CAD build for the part. Positions are in the model's coordinates, mm. A direction names the side the tool comes from. Coordinates: 2 decimals unless noted, no trailing zeros. Loops run counter-clockwise (first coordinate to the right, second up) from the corner with the lowest first, then second, coordinate; pieces in that order, holes last. Notation, with made-up numbers: (2, 27) -> (40, 27) arc R23 ccw to (40, 61) -> close; hole circle Ø6 at (28, 69.25). An arc over 180 degrees is marked (long way). Answer as CSV lines item,"result". Start each with the question number.
```python
from build123d import *

# Parameters (mm, degrees)
BOSS_EXTRUDE1_DEPTH = 40
SKETCH2_R           = 2.5
CUT_EXTRUDE1_DEPTH  = 79.89866919


with BuildPart() as part:
    # Sketch1 → Boss-Extrude1 (new body)
    with BuildSketch(Plane(origin=(0, 0, 0), x_dir=(1, 0, 0), z_dir=(0, 1, 0))):
        Polygon((0, 0), (0, 20), (3, 20), (3, 3), (65, 3), (65, 0), align=None)
    extrude(amount=BOSS_EXTRUDE1_DEPTH)

    # Sketch2 → Cut-Extrude1 (cut, through all)
    with BuildSketch(Plane.XY):
        with Locations((21.15, 20)):
            Circle(SKETCH2_R)
        with Locations((57.65, 20)):
            Circle(SKETCH2_R)
    extrude(amount=-CUT_EXTRUDE1_DEPTH, mode=Mode.SUBTRACT)


solid = part.part
```
Q1. Saw through at B-B (x = 21.15). List the corners of the cut face in (y, z).
Q2. Probe probe 1 along Y at (x, z) = (21.15, -2.1); probe 2 along Z at (x, y) = (40, 9); probe 3 along X at (y, z) = (36, -11). List the from-to ranges inside material, lowest first. Write a range as from..to.
Q3. Which spindle directions (+Z, -Z, +X, -X, +Y, -Y) get a long thin tool onto all of the face, cutting with end or side? Do faces 4 (the flat face through (3, 20, -12)), 5 (the cylindrical face through (58.99, 22.11, -1.48)). Say none if no direction does.
Q4. Saw through at A-A (y = 20). List the corners of the cut face in (x, z).
Q5. Saw through at C-C (y = 12.5). List the corners of the cut face in (x, z), and give its area (3 significant figures).
Q6. Saw through at D-D (z = -6.5). List the corners of the cut face in (x, y), and give its area (3 significant figures).
Q7. Pin check, flat tips, straight feed: pin 1 Ø2 at (x, y) = (9, 32.5) entering from -Z; pin 2 Ø4 at (x, y) = (21.15, 20) entering from -Z; pin 3 Ø5 at (y, z) = (11.5, -9) entering from +X. Stop position of each tip, or through.
Q8. Two-plate mould, pull along Y, no slides. Class faces 1 (the flat face through (0, 20, -10)), 2 (the cylindrical face through (22.49, 22.11, -1.48)), 3 (the flat face through (28, 40, -2)): pulls with the +Y half, pulls with the -Y half, needs draft (parallel to the pull), parting line crosses it, or undercut.
Ans:
1,outline,"(0, -3) -> (17.5, -3) -> (17.5, 0) -> (0, 0) -> close; (22.5, -3) -> (40, -3) -> (40, 0) -> (22.5, 0) -> close"
2,probe 1,"y = 0..17.5, 22.5..40"
2,probe 2,"z = -3..0"
2,probe 3,"x = 0..3"
3,face 4,"-Z, +X, +Y, -Y"
3,face 5,"+Z, -Z"
4,outline,"(0, -20) -> (3, -20) -> (3, -3) -> (18.65, -3) -> (18.65, 0) -> (0, 0) -> close; (23.65, -3) -> (55.15, -3) -> (55.15, 0) -> (23.65, 0) -> close; (60.15, -3) -> (65, -3) -> (65, 0) -> (60.15, 0) -> close"
5,outline,"(0, -20) -> (3, -20) -> (3, -3) -> (65, -3) -> (65, 0) -> (0, 0) -> close"
5,area,"246 mm²"
6,outline,"(0, 0) -> (3, 0) -> (3, 40) -> (0, 40) -> close"
6,area,"120 mm²"
7,pin 1,"stops at z = -3"
7,pin 2,"passes through"
7,pin 3,"stops at x = 3"
8,face 1,"needs draft"
8,face 2,"undercut"
8,face 3,"pulls with the +Y half"
